Work out the finished part from the listing and answer in its coordinate system (mm). A direction names the side the tool comes from. Round coordinates to 2 decimals unless told otherwise and drop trailing zeros. Loops run counter-clockwise (first coordinate to the right, second up) from the corner with the lowest first, then second, coordinate; pieces in that order, holes last. Notation, with made-up numbers: (30, 64.5) - (48, 64.5) arc R27 cw to (48, 90.5) - close; hole circle Ø6 at (-11, 80.5). An arc over 180 degrees is marked (long way). Return JSON: item names as keys, results as strings.
from build123d import *

# Parameters (mm, degrees)
EXTRUDE_THIN1_DEPTH = 8


with BuildPart() as part:
    # Sketch1 → Extrude-Thin1 (new body)
    with BuildSketch(Plane(origin=(0, 0, 0), x_dir=(1, 0, 0), z_dir=(0, 1, 0))):
        with BuildLine():
            Line((-3.025, -6.2), (-3.025, -0.670820393))
            ThreePointArc((-3.025, -0.670820393), (-3.064643255, -0.551297532), (-3.167857143, -0.479157424))
            ThreePointArc((-3.167857143, -0.479157424), (-3.525, 0), (-3.167857143, 0.479157424))
            ThreePointArc((-3.167857143, 0.479157424), (-3.064643255, 0.551297532), (-3.025, 0.670820393))
            Line((-3.025, 0.670820393), (-3.025, 5.6))
            ThreePointArc((-3.025, 5.6), (-2.878553391, 5.953553391), (-2.525, 6.1))
            Line((-2.525, 6.1), (2.525, 6.1))
            ThreePointArc((2.525, 6.1), (2.878553391, 5.953553391), (3.025, 5.6))
            Line((3.025, 5.6), (3.025, 0.670820393))
            ThreePointArc((3.025, 0.670820393), (3.064643255, 0.551297532), (3.167857143, 0.479157424))
            ThreePointArc((3.167857143, 0.479157424), (3.525, 0), (3.167857143, -0.479157424))
            ThreePointArc((3.167857143, -0.479157424), (3.064643255, -0.551297532), (3.025, -0.670820393))
            Line((3.025, -0.670820393), (3.025, -6.2))
            Line((3.025, -6.2), (3.205, -6.2))
            Line((3.205, -6.2), (3.205, -0.670820393))
            ThreePointArc((3.205, -0.670820393), (3.208964325, -0.658868107), (3.219285714, -0.651654096))
            ThreePointArc((3.219285714, -0.651654096), (3.705, 0), (3.219285714, 0.651654096))
            ThreePointArc((3.219285714, 0.651654096), (3.208964325, 0.658868107), (3.205, 0.670820393))
            Line((3.205, 0.670820393), (3.205, 5.6))
            ThreePointArc((3.205, 5.6), (3.005832611, 6.080832611), (2.525, 6.28))
            Line((2.525, 6.28), (-2.525, 6.28))
            ThreePointArc((-2.525, 6.28), (-3.005832611, 6.080832611), (-3.205, 5.6))
            Line((-3.205, 5.6), (-3.205, 0.670820393))
            ThreePointArc((-3.205, 0.670820393), (-3.208964325, 0.658868107), (-3.219285714, 0.651654096))
            ThreePointArc((-3.219285714, 0.651654096), (-3.705, 0), (-3.219285714, -0.651654096))
            ThreePointArc((-3.219285714, -0.651654096), (-3.208964325, -0.658868107), (-3.205, -0.670820393))
            Line((-3.205, -0.670820393), (-3.205, -6.2))
            Line((-3.205, -6.2), (-3.025, -6.2))
        make_face()
    extrude(amount=EXTRUDE_THIN1_DEPTH)


solid = part.part
1) Find the intervals of material crossed by L1, parallel to X at y = 6, z = 4.5 (3 decimals); L2, parallel to Z at x = -0.5, y = 2; L3, parallel to Z at x = 3.25, y = 3.5, in increasing order.
Verdict:
{"L1": "x = -3.205 to -3.025, 3.025 to 3.205", "L2": "z = -6.28 to -6.1", "L3": "z = -0.64 to -0.45, 0.45 to 0.64"}
2) Section A-A (z = 3.25) is taken. Give the vertices of the cut face in (x, y) (3 decimals).
Verdict:
{"outline": "(-3.205, 0) - (-3.025, 0) - (-3.025, 8) - (-3.205, 8) - close; (3.025, 0) - (3.205, 0) - (3.205, 8) - (3.025, 8) - close"}
3) Flat-ended cylindrical pins translate along their axes: pin 1 (4 mm diameter, centred on y = 5.5, z = -3, fed in from +X) (3 decimals); pin 2 (3 mm diameter, centred on y = 6, z = 3.5, fed in from -X) (3 decimals); pin 3 (1.5 mm diameter, centred on x = 1, y = 6, fed in from +Z). Find the tip coordinate at first contact, or state that the pin passes through.
Verdict:
{"pin 1": "stops at x = 3.205", "pin 2": "stops at x = -3.205", "pin 3": "stops at z = -6.1"}
4) A tool of negligible diameter and unlimited length cuts with its end or side. For faces 1 (the flat face through (-3.205, 4, -3)), 2 (the flat face through (3.205, 4, 3)), 3 (the flat face through (-3.025, 4, -3)), 4 (the cylindrical face through (-3.525, 3.944, 0.009)), from which of +Z, -Z, +X, -X, +Y, -Y can it reach the whole face along a straight path? Write none if from no direction.
Verdict:
{"face 1": "-Z, -X, +Y, -Y", "face 2": "+Z, +X, +Y, -Y", "face 3": "+Z, +Y, -Y", "face 4": "+Y, -Y"}
5) Section D-D (x = -0.25) is taken. Give the vertices of the cut face in (y, z).
Verdict:
{"outline": "(0, -6.28) - (8, -6.28) - (8, -6.1) - (0, -6.1) - close"}
6) Section C-C (z = 0.25) is taken. Give the vertices of the cut face in (x, y).
Verdict:
{"outline": "(-3.66, 0) - (-3.46, 0) - (-3.46, 8) - (-3.66, 8) - close; (3.46, 0) - (3.66, 0) - (3.66, 8) - (3.46, 8) - close"}
7) Determine the mould class of faces 5 (the flat face through (-3.025, 4, 3)), 6 (the flat face through (0, 4, -6.28)), 7 (the flat face through (-3.205, 4, 3)) for opening direction X: pulls with the +X half, pulls with the -X half, needs draft (parallel to the pull), parting line crosses it, or undercut.
Verdict:
{"face 5": "undercut", "face 6": "needs draft", "face 7": "pulls with the -X half"}
8) Section B-B (y = 5) is taken. Give the vertices of the cut face in (x, z) (3 decimals), and give its area (3 significant figures).
Verdict:
{"outline": "(-3.219, -0.652) arc R0.02 cw to (-3.205, -0.671) - (-3.205, -5.6) arc R0.68 ccw to (-2.525, -6.28) - (2.525, -6.28) arc R0.68 ccw to (3.205, -5.6) - (3.205, -0.671) arc R0.02 cw to (3.219, -0.652) arc R0.68 ccw to (3.219, 0.652) arc R0.02 cw to (3.205, 0.671) - (3.205, 6.2) - (3.025, 6.2) - (3.025, 0.671) arc R0.2 ccw to (3.168, 0.479) arc R0.5 cw to (3.168, -0.479) arc R0.2 ccw to (3.025, -0.671) - (3.025, -5.6) arc R0.5 cw to (2.525, -6.1) - (-2.525, -6.1) arc R0.5 cw to (-3.025, -5.6) - (-3.025, -0.671) arc R0.2 ccw to (-3.168, -0.479) arc R0.5 cw to (-3.168, 0.479) arc R0.2 ccw to (-3.025, 0.671) - (-3.025, 6.2) - (-3.205, 6.2) - (-3.205, 0.671) arc R0.02 cw to (-3.219, 0.652) arc R0.68 ccw to start", "area": "5.65 mm2"}
